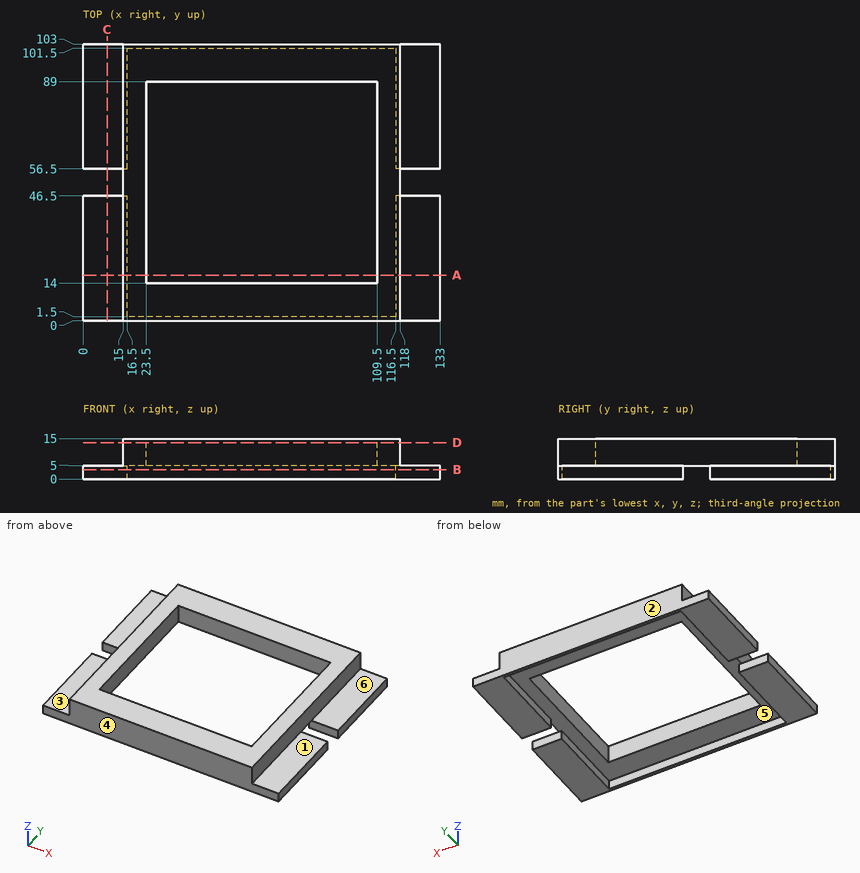
For this review, use the dimensioned drawing (mm, ordinates from the lowest corner) and the shaded views. A direction names the side the tool comes from. Coordinates: 2 decimals unless noted, no trailing zeros. Loops run counter-clockwise (first coordinate to the right, second up) from the corner with the lowest first, then second, coordinate; pieces in that order, holes last. Notation, with made-up numbers: (-18.75, -39.5) -> (27.25, -39.5) arc R11 cw to (27.25, -32.5) -> close; hole circle Ø1 at (71.25, 45). An arc over 180 degrees is marked (long way). Write each question's results on one line, items separated by ' | '.
Q1. To check wall thickness, follow line 1 along Y through (x, z) = (105.5, 5.75); line 2 along X through (y, z) = (42.5, 12.5); line 3 along X through (y, z) = (79, 3.5). State the ranges of each line that lie inside material, in increasing order. Write a range as [from, to].
Taken from the geometry:
line 1: [0, 14], [89, 103] | line 2: [15, 23.5], [109.5, 118] | line 3: [0, 16.5], [116.5, 133]
Q2. Add section B-B, the plane z = 3.5. State the section outline as (x, y) points, then the cut area to 3 significant figures.
Taken from the geometry:
outline: (0, 0) -> (133, 0) -> (133, 46.5) -> (116.5, 46.5) -> (116.5, 1.5) -> (16.5, 1.5) -> (16.5, 46.5) -> (0, 46.5) -> close; (0, 56.5) -> (16.5, 56.5) -> (16.5, 101.5) -> (116.5, 101.5) -> (116.5, 56.5) -> (133, 56.5) -> (133, 103) -> (0, 103) -> close | area: 3,370 mm²
Q3. Machinability: for the marked faces 1, 2 and 3, which of the approach directions +Z, -Z, +X, -X, +Y, -Y give a long, thin tool a straight path to every point of the face, cutting with its end or side? Answer none if there is none.
Taken from the geometry:
face 1: +Z, +X, +Y, -Y | face 2: +Z, -Z, +X, -X, +Y | face 3: +Z, -X, +Y, -Y
Q4. Mouldability with a two-part tool opening along Y and no side actions: class the marked faces 4, 5 and 6 as +Y half, -Y half, draft (parallel to the pull), parting line (faces both ways), or undercut.
Taken from the geometry:
face 4: -Y half | face 5: undercut | face 6: draft
Q5. Add section C-C, the plane x = 9. State the section outline as (y, z) points, then the cut area to 3 significant figures.
Taken from the geometry:
outline: (0, 0) -> (46.5, 0) -> (46.5, 5) -> (0, 5) -> close; (56.5, 0) -> (103, 0) -> (103, 5) -> (56.5, 5) -> close | area: 465 mm²
Q6. Add section A-A, the plane y = 17. State the section outline as (x, z) points, then the cut area to 3 significant figures.
Taken from the geometry:
outline: (0, 0) -> (16.5, 0) -> (16.5, 5) -> (23.5, 5) -> (23.5, 15) -> (15, 15) -> (15, 5) -> (0, 5) -> close; (109.5, 5) -> (116.5, 5) -> (116.5, 0) -> (133, 0) -> (133, 5) -> (118, 5) -> (118, 15) -> (109.5, 15) -> close | area: 335 mm²
Q7. Add section D-D, the plane z = 13.5. State the section outline as (x, y) points.
Taken from the geometry:
outline: (15, 0) -> (118, 0) -> (118, 103) -> (15, 103) -> close; hole (23.5, 14) -> (109.5, 14) -> (109.5, 89) -> (23.5, 89) -> close
Q8. For pin 1 Ø7.5 at (x, y) = (9, 26.5) entering from +Z; pin 2 Ø5 at (y, z) = (53, 10.5) entering from -X; pin 3 Ø3 at (y, z) = (60.5, 11) entering from +X, all flat-tipped, find the tip position at first contact; note any pin that passes through.
Taken from the geometry:
pin 1: z = 5 | pin 2: x = 15 | pin 3: x = 118
